Could you check a few things on this model? Use its own coordinates, in mm. Face numbers are marked on the shaded views. Coordinates: 2 decimals unless noted, no trailing zeros. Write each loop counter-clockwise with the first axis right and the second up, starting at its lowest first coordinate (ties: lowest second). Pieces come first, ordered by that corner, then holes. Notation, with made-up numbers: M 58.25,9 L 83.25,9 A20 ccw 83.25,21 Z; hole C 73,56.5 d11. An arc over 180 degrees is marked long. Write item = value, one per line.
```python
from build123d import *

# Parameters (mm, degrees)
SKETCH_1_R          = 17.5
SKETCH_1_R_2        = 10
EXTRUDE_1_DEPTH     = 20
SKETCH_2_W          = 0.5
SKETCH_2_H          = 19.301562603
CUT_EXTRUDE_1_DEPTH = 15
SKETCH_3_W          = 0.5
SKETCH_3_H          = 20.813345434
CUT_EXTRUDE_2_DEPTH = 15


with BuildPart() as part:
    # 草图1 → 凸台-拉伸1 (new body)
    with BuildSketch(Plane.XY):
        Circle(SKETCH_1_R)
        Circle(SKETCH_1_R_2, mode=Mode.SUBTRACT)
    extrude(amount=EXTRUDE_1_DEPTH)

    # 草图2 → 切除-拉伸1 (cut)
    with BuildSketch(Plane.XY.offset(20)):
        with Locations((-1.195478964, -9.928284345)):
            Rectangle(SKETCH_2_W, SKETCH_2_H)
    extrude(amount=-CUT_EXTRUDE_1_DEPTH, mode=Mode.SUBTRACT)

    # 草图3 → 切除-拉伸2 (cut)
    with BuildSketch(Plane(origin=(0, 0, 0), x_dir=(-1, 0, 0), z_dir=(0, 0, -1))):
        with Locations((-0.669659449, 7.720299062)):
            Rectangle(SKETCH_3_W, SKETCH_3_H)
    extrude(amount=-CUT_EXTRUDE_2_DEPTH, mode=Mode.SUBTRACT)


solid = part.part
```
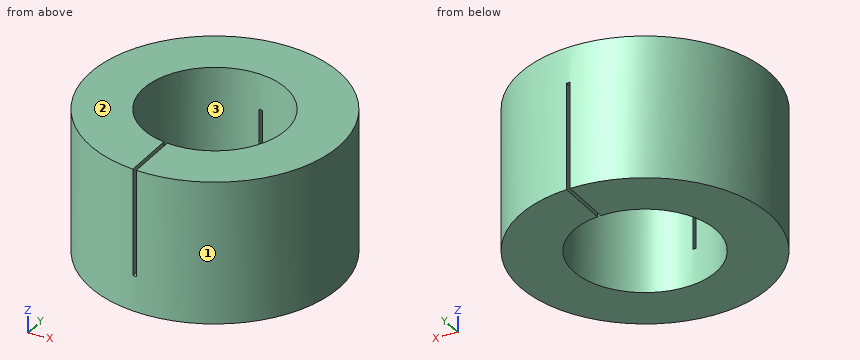
Item 1: Imagine slicing it at B-B (y = 0). Write out the boundary of the cut face in (x, z).
Numbers:
outline = M -17.5,0 L -10,0 L -10,20 L -17.5,20 Z; M 10,0 L 17.5,0 L 17.5,20 L 10,20 Z
Item 2: I'm going to push flat-ended pins straight in: P1, Ø6, axis at y = 14, z = 4.5, coming from the -X side; P2, Ø4, axis at x = -7.5, z = 4, coming from the -Y side; P3, Ø2.5, axis at y = 13, z = 8.5, coming from the +X side; P4, Ø8, axis at x = -1.5, y = 4, coming from the +Z side. Where does each tip first touch, or does it pass through?
Numbers:
P1 = -13.61
P2 = -16.61
P3 = 12.97
P4 = through
Item 3: Imagine slicing it at D-D (z = 4.25). Write out the boundary of the cut face in (x, y).
Numbers:
outline = M 0.42,9.99 L 0.42,17.49 A17.5 ccw long 0.92,17.48 L 0.92,9.96 A10 cw long Z
Item 4: Imagine slicing it at A-A (z = 14). Write out the boundary of the cut face in (x, y).
Numbers:
outline = M -1.45,-17.44 L -1.45,-9.89 A10 cw 0.42,9.99 L 0.42,17.49 A17.5 ccw Z; M -0.95,-17.47 A17.5 ccw 0.92,17.48 L 0.92,9.96 A10 cw -0.95,-9.96 Z
Item 5: If I drill on line 1 along Y through (x, z) = (0, 8.5); line 2 along X through (y, z) = (-1, 16.25), over which ranges is the centre line in solid material (lowest first)?
Numbers:
line_1 = -17.5 to -10, 10 to 17.5
line_2 = -17.47 to -9.95, 9.95 to 17.47
Item 6: If we mould it in two halves opening along X, with no side actions, what happens to the marked faces 1, 2 and 3? For each: pulls with the +X half, pulls with the -X half, needs draft (parallel to the pull), parting line crosses it, or undercut.
Numbers:
face_1 = parting line crosses it
face_2 = needs draft
face_3 = undercut
Item 7: Imagine slicing it at C-C (y = 11). Write out the boundary of the cut face in (x, z).
Numbers:
outline = M -13.61,0 L 0.42,0 L 0.42,15 L 0.92,15 L 0.92,0 L 13.61,0 L 13.61,20 L -13.61,20 Z
